from build123d import *

# Parameters (mm, degrees)
F2_DEPTH = 2.5


with BuildPart() as f2:
    # F1 (on Front) → F2 (new body, symmetric)
    with BuildSketch(Plane.XZ):
        with BuildLine():
            Line((-13.65, -9.118186), (-14.15, -9.118186))
            ThreePointArc((-14.15, -9.118186), (-14.857107, -9.41108), (-15.15, -10.118186))
            ThreePointArc((-15.15, -10.118186), (-14.857107, -10.825293), (-14.15, -11.118186))
            Line((-14.15, -11.118186), (-11.15, -11.118186))
            ThreePointArc((-11.15, -11.118186), (-10.442893, -10.825293), (-10.15, -10.118186))
            Line((-10.15, -10.118186), (-10.15, -8.118186))
            ThreePointArc((-10.15, -8.118186), (-9.857107, -7.41108), (-9.15, -7.118186))
            Line((-9.15, -7.118186), (0, -7.118186))
            Line((0, -7.118186), (0, -4.742948))
            Line((0, -4.742948), (-7, -4.742948))
            Line((-7, -4.742948), (-7, -1.342948))
            ThreePointArc((-7, -1.342948), (-6.469822, 0.815107), (-5, 2.481814))
            Line((-5, 2.481814), (-5, 3.875005))
            ThreePointArc((-5, 3.875005), (-11.136524, 1.120804), (-13.65, -5.118186))
            Line((-13.65, -5.118186), (-13.65, -9.118186))
        make_face()
    extrude(amount=F2_DEPTH, both=True)

    # F3: F2 across face


with BuildPart() as f2_1:
    add(f2.part)
    add(f2.part.mirror(Plane(origin=(0, 0, -5.930567), x_dir=(0, 1, 0), z_dir=(1, 0, 0))))


solid = f2_1.part
The model under review builds one solid part; all positions refer to its coordinate system, in mm. A direction names the side the tool comes from. Coordinates: 2 decimals unless noted, no trailing zeros. Order: outer loops, then holes, each group sorted by start corner. A loop starts at its lowest first (then second) coordinate and runs counter-clockwise, first axis right, second up. Notation, with made-up numbers: (2.25, 62.5) -> (47.25, 62.5) arc R35 cw to (47.25, 94.5) -> close; hole circle Ø7 at (41.5, 33.5). An arc over 180 degrees is marked (long way). Answer in a Markdown table with one row per item.
(1) Consider section B-B (y = -0.7). Write out the cut boundary in (x, z) (3 decimals), plus the area to 3 significant figures.
Answers:
| item | result |
|---|---|
| outline | (-15.15, -10.118) arc R1 ccw to (-14.15, -11.118) -> (-11.15, -11.118) arc R1 ccw to (-10.15, -10.118) -> (-10.15, -8.118) arc R1 cw to (-9.15, -7.118) -> (9.15, -7.118) arc R1 cw to (10.15, -8.118) -> (10.15, -10.118) arc R1 ccw to (11.15, -11.118) -> (14.15, -11.118) arc R1 ccw to (15.15, -10.118) arc R1 ccw to (14.15, -9.118) -> (13.65, -9.118) -> (13.65, -5.118) arc R9 ccw to (5, 3.875) -> (5, 2.482) arc R4.657 cw to (7, -1.343) -> (7, -4.743) -> (-7, -4.743) -> (-7, -1.343) arc R4.657 cw to (-5, 2.482) -> (-5, 3.875) arc R9 ccw to (-13.65, -5.118) -> (-13.65, -9.118) -> (-14.15, -9.118) arc R1 ccw to start |
| area | 188 mm² |
(2) The part is to be moulded in two halves that separate along Z. For faces 5 (the flat face through (-7, 0, -3)), 6 (the cylindrical face through (11.07, -0.04, 1.19)), 7 (the flat face through (-13.65, 0, -7)), say which applies: +Z half, -Z half, draft (parallel to the pull), parting line (faces both ways), or undercut.
Answers:
| item | result |
|---|---|
| face 5 | undercut |
| face 6 | +Z half |
| face 7 | draft |
(3) Wall thickness on line 1 along X through (y, z) = (1.75, -8.75); line 2 along Z through (x, y) = (14, -1.8); line 3 along X through (y, z) = (2.05, -4): over which ranges is each line inside the solid? List them lowest first.
Answers:
| item | result |
|---|---|
| line 1 | -13.65 to -10.15, 10.15 to 13.65 |
| line 2 | -11.12 to -9.12 |
| line 3 | -13.58 to -7, 7 to 13.58 |
(4) Insertion check: pin 1 (2 mm diameter, centred on y = 0, z = -6.5, fed in from +X); pin 2 (2.5 mm diameter, centred on y = -1, z = -3, fed in from -X); pin 3 (1.1 mm diameter, centred on y = 1, z = 3, fed in from +X). Each pin has a flat end and moves straight along its axis. Give the tip position at first contact, or say it passes through.
Answers:
| item | result |
|---|---|
| pin 1 | x = 13.65 |
| pin 2 | x = -13.61 |
| pin 3 | x = 9.52 |
(5) Consider section C-C (x = 1). Write out the cut boundary in (y, z).
Answers:
| item | result |
|---|---|
| outline | (-2.5, -7.12) -> (2.5, -7.12) -> (2.5, -4.74) -> (-2.5, -4.74) -> close |
(6) Consider section A-A (z = -3.5). Write out the cut boundary in (x, y).
Answers:
| item | result |
|---|---|
| outline | (-13.5, -2.5) -> (-7, -2.5) -> (-7, 2.5) -> (-13.5, 2.5) -> close; (7, -2.5) -> (13.5, -2.5) -> (13.5, 2.5) -> (7, 2.5) -> close |
(7) Machinability: for faces 1 (the flat face through (13.65, 0, -7)), 2 (the cylindrical face through (-6.484, -0.035, 0.787)), 3 (the flat face through (-5, 0, 3)), 4 (the flat face through (10.15, 0, -9)), which of the approach directions +Z, -Z, +X, -X, +Y, -Y give a long, thin tool a straight path to every point of the face, cutting with its end or side? Answer none if there is none.
Answers:
| item | result |
|---|---|
| face 1 | +Z, +X, +Y, -Y |
| face 2 | +Y, -Y |
| face 3 | +Z, +Y, -Y |
| face 4 | -Z, +Y, -Y |
(8) Consider section D-D (z = -6.5). Write out the cut boundary in (x, y).
Answers:
| item | result |
|---|---|
| outline | (-13.65, -2.5) -> (13.65, -2.5) -> (13.65, 2.5) -> (-13.65, 2.5) -> close |
